Work out the finished part from the listing and answer in its coordinate system (mm). A direction names the side the tool comes from. Give positions to 0.01 mm unless a question says otherwise; leave off trailing zeros. Loops run counter-clockwise (first coordinate to the right, second up) from the corner with the lowest first, then second, coordinate; pieces in that order, holes last. Notation, with made-up numbers: M 29,10 L 55,10 A22 cw 55,43 Z; hole C 82.5,-9.5 d5. An arc over 180 degrees is marked long. Use a Markdown table: item, result.
```python
from build123d import *

# Parameters (mm, degrees)
BOSS_EXTRUDE1_DEPTH                             = 19.05
CSK_FOR_M6_FLAT_HEAD_MACHINE_SCREW1_D           = 6.6
CSK_FOR_M6_FLAT_HEAD_MACHINE_SCREW1_CSINK_D     = 12.6
CSK_FOR_M6_FLAT_HEAD_MACHINE_SCREW1_CSINK_ANGLE = 90
CSK_FOR_M6_FLAT_HEAD_MACHINE_SCREW2_D           = 6.6
CSK_FOR_M6_FLAT_HEAD_MACHINE_SCREW2_CSINK_D     = 12.6
CSK_FOR_M6_FLAT_HEAD_MACHINE_SCREW2_CSINK_ANGLE = 90


with BuildPart() as part:
    # Sketch1 → Boss-Extrude1 (new, symmetric)
    with BuildSketch(Plane.XY):
        Polygon((0, 4.567772054), (0, 0), (4.567772054, 0), (38.1, 0), (38.1, 6.35), (6.35, 6.35), (6.35, 38.1), (0, 38.1), align=None)
    extrude(amount=BOSS_EXTRUDE1_DEPTH, both=True)

    # CSK for M6 Flat Head Machine Screw1 (through all)
    with Locations(Plane(origin=(6.35, 0, 0), x_dir=(0, 0, -1), z_dir=(1, 0, 0))):
        with Locations((0, 25.4)):
            CounterSinkHole(CSK_FOR_M6_FLAT_HEAD_MACHINE_SCREW1_D / 2, CSK_FOR_M6_FLAT_HEAD_MACHINE_SCREW1_CSINK_D / 2, counter_sink_angle=CSK_FOR_M6_FLAT_HEAD_MACHINE_SCREW1_CSINK_ANGLE)

    # CSK for M6 Flat Head Machine Screw2 (through all)
    with Locations(Plane(origin=(0, 6.35, 0), x_dir=(1, 0, 0), z_dir=(0, 1, 0))):
        with Locations((25.4, 0)):
            CounterSinkHole(CSK_FOR_M6_FLAT_HEAD_MACHINE_SCREW2_D / 2, CSK_FOR_M6_FLAT_HEAD_MACHINE_SCREW2_CSINK_D / 2, counter_sink_angle=CSK_FOR_M6_FLAT_HEAD_MACHINE_SCREW2_CSINK_ANGLE)


solid = part.part
```
(1) A cutting plane is placed at D-D (y = 5). Write down the section's boundary in (x, z).
Entries:
| item | result |
|---|---|
| outline | M 0,-19.05 L 38.1,-19.05 L 38.1,19.05 L 0,19.05 Z; hole C 25.4,0 d9.9 |
(2) A cutting plane is placed at A-A (z = 0). Write down the section's boundary in (x, y), and give its area (3 significant figures).
Entries:
| item | result |
|---|---|
| outline | M 0,0 L 22.1,0 L 22.1,3.35 L 19.1,6.35 L 6.35,6.35 L 6.35,19.1 L 3.35,22.1 L 0,22.1 Z; M 0,28.7 L 3.35,28.7 L 6.35,31.7 L 6.35,38.1 L 0,38.1 Z; M 28.7,0 L 38.1,0 L 38.1,6.35 L 31.7,6.35 L 28.7,3.35 Z |
| area | 342 mm² |
(3) The mould has two halves that part along Z. Classify faces 3 (the flat face through (6, 13, 19.05)), 4 (the conical face through (28.842, 3.496, -0.151)), 5 (the flat face through (0, 19, 0)): released by +Z, released by -Z, zero draft, split by the parting line, or undercut.
Entries:
| item | result |
|---|---|
| face 3 | released by +Z |
| face 4 | undercut |
| face 5 | zero draft |
(4) A cutting plane is placed at B-B (y = 25.4). Write down the section's boundary in (x, z).
Entries:
| item | result |
|---|---|
| outline | M 0,-19.05 L 6.35,-19.05 L 6.35,-6.3 L 3.35,-3.3 L 0,-3.3 Z; M 0,3.3 L 3.35,3.3 L 6.35,6.3 L 6.35,19.05 L 0,19.05 Z |
(5) Consider probe 1 along Y at (x, z) = (2.5, 0); probe 2 along Z at (x, y) = (25.4, 1.7); probe 3 along Y at (x, z) = (23, -12.5). Determine where each line is inside the solid, lowest interval first. Write a range as [from, to].
Entries:
| item | result |
|---|---|
| probe 1 | y = [0, 22.1], [28.7, 38.1] |
| probe 2 | z = [-19.05, -3.3], [3.3, 19.05] |
| probe 3 | y = [0, 6.35] |
(6) Which of the six approach directions +Z, -Z, +X, -X, +Y, -Y give full straight-line access (tool end or side, diameter ignored) to faces 1 (the flat face through (18.9, 6.35, 0.3)), 2 (the conical face through (3.5, 28.82, -0.45))?
Entries:
| item | result |
|---|---|
| face 1 | +Z, -Z, +X, +Y |
| face 2 | +X |
